from build123d import *

# Parameters (mm, degrees)
SKETCH2_W                    = 80
SKETCH2_H                    = 41
BOSS_EXTRUDE1_DEPTH          = 68
FILLET1_R                    = 3
SKETCH5_OUTSIDE_W            = 104.544
SKETCH5_OUTSIDE_H            = 65.544
CUT_EXTRUDE2_DEPTH           = 48
CUT_EXTRUDE3_DEPTH           = 82.672987579
FILLET2_R                    = 3
FILLET3_R                    = 3
M10_TAPPED_HOLE1_D           = 8.5
M10_TAPPED_HOLE1_DEPTH       = 16.946342369
M10_TAPPED_HOLE1_CSINK_D     = 10.05
M10_TAPPED_HOLE1_CSINK_ANGLE = 90
M10_TAPPED_HOLE1_TIP         = 2.553657631


with BuildPart() as part:
    # Sketch2 → Boss-Extrude1 (new body)
    with BuildSketch(Plane(origin=(0, 0, 0), x_dir=(1, 0, 0), z_dir=(0, 1, 0))):
        with Locations((0, -0.63)):
            Rectangle(SKETCH2_W, SKETCH2_H)
    extrude(amount=-BOSS_EXTRUDE1_DEPTH)

    # Fillet1
    fillet1_edges = [part.edges().sort_by_distance(p)[0] for p in [
        (40, -34, 21.13),
        (-40, -34, 21.13),
        (-40, -34, -19.87),
        (40, -34, -19.87),
    ]]
    fillet(fillet1_edges, radius=FILLET1_R)

    # Sketch5 outside → Cut-Extrude2 (cut)
    with BuildSketch(Plane.XZ.offset(68)):
        with Locations((0, 0.63)):
            Rectangle(SKETCH5_OUTSIDE_W, SKETCH5_OUTSIDE_H)
        with BuildLine():
            Line((19, -19.87), (24, -19.87))
            Line((24, -19.87), (24, 21.13))
            Line((24, 21.13), (-24, 21.13))
            Line((-24, 21.13), (-24, -19.87))
            Line((-24, -19.87), (-19, -19.87))
            Line((-19, -19.87), (-19, -14.37))
            ThreePointArc((-19, -14.37), (-17.242640687, -10.127359313), (-13, -8.37))
            Line((-13, -8.37), (-9, -8.37))
            ThreePointArc((-9, -8.37), (-6.878679656, -7.491320344), (-6, -5.37))
            Line((-6, -5.37), (-6, 10.13))
            ThreePointArc((-6, 10.13), (0, 16.13), (6, 10.13))
            Line((6, 10.13), (6, -5.37))
            ThreePointArc((6, -5.37), (6.878679656, -7.491320344), (9, -8.37))
            Line((9, -8.37), (13, -8.37))
            ThreePointArc((13, -8.37), (17.242640687, -10.127359313), (19, -14.37))
            Line((19, -14.37), (19, -19.87))
        make_face(mode=Mode.SUBTRACT)
    extrude(amount=-CUT_EXTRUDE2_DEPTH, mode=Mode.SUBTRACT)

    # Sketch6 → Cut-Extrude3 (cut, through all)
    with BuildSketch(Plane.XZ.offset(68)):
        with BuildLine():
            Line((-13, -8.37), (-9, -8.37))
            ThreePointArc((-9, -8.37), (-6.878679656, -7.491320344), (-6, -5.37))
            Line((-6, -5.37), (-6, 10.13))
            ThreePointArc((-6, 10.13), (0, 16.13), (6, 10.13))
            Line((6, 10.13), (6, -5.37))
            ThreePointArc((6, -5.37), (6.878679656, -7.491320344), (9, -8.37))
            Line((9, -8.37), (13, -8.37))
            ThreePointArc((13, -8.37), (17.242640687, -10.127359313), (19, -14.37))
            Line((19, -14.37), (19, -19.87))
            Line((19, -19.87), (-19, -19.87))
            Line((-19, -19.87), (-19, -14.37))
            ThreePointArc((-19, -14.37), (-17.242640687, -10.127359313), (-13, -8.37))
        make_face()
    extrude(amount=-CUT_EXTRUDE3_DEPTH, mode=Mode.SUBTRACT)

    # Fillet2
    fillet2_edges = [part.edges().sort_by_distance(p)[0] for p in [
        (24, -44, 21.13),
        (-24, -44, 21.13),
    ]]
    fillet(fillet2_edges, radius=FILLET2_R)

    # Fillet3
    # the kernel refuses this fillet: 3 mm, written as the material it adds along each edge
    with BuildSketch(Plane(origin=(24, -20, -19.87), x_dir=(0, -1, 0), z_dir=(0, 0, 1)), Plane(origin=(-24, -20, 18.13), x_dir=(0, -1, 0), z_dir=(0, 0, -1))) as fillet3_piece_1:
        with BuildLine():
            CenterArc((FILLET3_R, FILLET3_R), FILLET3_R, 180, 90)
            Line((0, FILLET3_R), (0, 0))
            Line((0, 0), (FILLET3_R, 0))
        make_face()
    extrude(amount=38)
    with BuildSketch(Plane(origin=(-21, -20, 18.13), x_dir=(0.5976672776328279, 0, -0.801744239297648), z_dir=(-0.801744239297648, 0, -0.5976672776328279))) as fillet3_piece_2_section:
        with BuildLine():
            CenterArc((3 + FILLET3_R, FILLET3_R), FILLET3_R, 180, 90)
            Line((3 + FILLET3_R, 0), (3, 0))
            Line((3, 0), (3, FILLET3_R))
        make_face()
    fillet3_piece_2 = revolve(axis=Axis((-21, -20, 18.13), (0, -1, 0)), revolution_arc=233.296989237, mode=Mode.PRIVATE)
    fillet3_piece_2 = split(fillet3_piece_2, bisect_by=Plane(origin=(-23.249816778, -20.934885373, 21.13), z_dir=(0, 0, -1)), keep=Keep.TOP, mode=Mode.PRIVATE)
    add(fillet3_piece_2)
    with BuildSketch(Plane(origin=(21, -20, 18.13), x_dir=(-0.5976672776328279, 0, -0.801744239297648), z_dir=(0.801744239297648, 0, -0.5976672776328279))) as fillet3_piece_3_section:
        with BuildLine():
            CenterArc((3 + FILLET3_R, -FILLET3_R), FILLET3_R, 90, 90)
            Line((3, -FILLET3_R), (3, 0))
            Line((3, 0), (3 + FILLET3_R, 0))
        make_face()
    fillet3_piece_3 = revolve(axis=Axis((21, -20, 18.13), (0, 1, 0)), revolution_arc=233.296989237, mode=Mode.PRIVATE)
    fillet3_piece_3 = split(fillet3_piece_3, bisect_by=Plane(origin=(23.249816872, -20.934884795, 21.13), z_dir=(0, 0, -1)), keep=Keep.TOP, mode=Mode.PRIVATE)
    add(fillet3_piece_3)

    # M10 Tapped Hole1
    with Locations(Plane(origin=(0, 0, 0), x_dir=(1, 0, 0), z_dir=(0, 1, 0))):
        with Locations((27.5, -0.63), (-27.5, -0.63)):
            CounterSinkHole(M10_TAPPED_HOLE1_D / 2, M10_TAPPED_HOLE1_CSINK_D / 2, depth=M10_TAPPED_HOLE1_DEPTH, counter_sink_angle=M10_TAPPED_HOLE1_CSINK_ANGLE)
            with Locations((0, 0, -(M10_TAPPED_HOLE1_DEPTH + M10_TAPPED_HOLE1_TIP / 2))):  # 118° drill point
                Cone(0, M10_TAPPED_HOLE1_D / 2, M10_TAPPED_HOLE1_TIP, mode=Mode.SUBTRACT)


solid = part.part
Check sheet for the modelled part. Datum: model origin and axes. Units: mm. A direction names the side the tool comes from. Round coordinates to 2 decimals unless told otherwise and drop trailing zeros. Write each loop counter-clockwise with the first axis right and the second up, starting at its lowest first coordinate (ties: lowest second). Pieces come first, ordered by that corner, then holes. Notation, with made-up numbers: (-39.75, 62) - (-4.75, 62) arc R13 cw to (-4.75, 73) - close; hole circle Ø10 at (13.5, -26.75). An arc over 180 degrees is marked (long way). Return JSON: item names as keys, results as strings.
Q1. Scan lines: L1, parallel to Z at x = 27.5, y = -6; L2, parallel to X at y = -39.5, z = 4; L3, parallel to X at y = -3.5, z = -15. Record each from-to range of solid material in increasing order. Write a range as from..to.
Returned:
{"L1": "z = -19.87..-3.62, 4.88..21.13", "L2": "x = -24..-6, 6..24", "L3": "x = -40..-19, 19..40"}
Q2. Depth check by flat-ended pin: P1, Ø2, axis at x = 10.5, y = -50.5, coming from the -Z side; P2, Ø19, axis at y = -54, z = 2.5, coming from the +X side; P3, Ø3, axis at y = -32, z = 5.5, coming from the -X side. Enter the tip coordinate at first touch or a pass-through.
Returned:
{"P1": "stops at z = -8.37", "P2": "stops at x = 24", "P3": "stops at x = -24"}
Q3. Cross-section at C-C (y = -43.5). Record the boundary of the cut face in (x, z).
Returned:
{"outline": "(-24, -19.87) - (-19, -19.87) - (-19, -14.37) arc R6 cw to (-13, -8.37) - (-9, -8.37) arc R3 ccw to (-6, -5.37) - (-6, 10.13) arc R6 cw to (6, 10.13) - (6, -5.37) arc R3 ccw to (9, -8.37) - (13, -8.37) arc R6 cw to (19, -14.37) - (19, -19.87) - (24, -19.87) - (24, 18.13) arc R3 ccw to (21, 21.13) - (-21, 21.13) arc R3 ccw to (-24, 18.13) - close"}
Q4. Draft check along X on faces 1 (the cylindrical face through (-24.9, -20.86, -0.6)), 2 (the cylindrical face through (23.1, -45.18, 20.27)), 3 (the cylindrical face through (-23.254, -8.974, 0.443)), 4 (the cylindrical face through (-0.13, -34.48, 16.13)). Enter one of: released by +X, released by -X, zero draft, split by the parting line, or undercut.
Returned:
{"face 1": "released by -X", "face 2": "released by +X", "face 3": "undercut", "face 4": "undercut"}
Q5. Cross-section at D-D (x = 11). Record the boundary of the cut face in (y, z).
Returned:
{"outline": "(-68, -8.37) - (0, -8.37) - (0, 21.13) - (-68, 21.13) - close"}
Q6. Cross-section at A-A (z = 7). Record the boundary of the cut face in (x, y).
Returned:
{"outline": "(-40, -20) - (-27, -20) arc R3 cw to (-24, -23) - (-24, -68) - (-6, -68) - (-6, 0) - (-40, 0) - close; (6, -68) - (24, -68) - (24, -23) arc R3 cw to (27, -20) - (40, -20) - (40, 0) - (6, 0) - close"}
Q7. Cross-section at B-B (y = -8). Record the boundary of the cut face in (x, z), then the cut area to 3 significant figures.
Returned:
{"outline": "(-40, -16.87) arc R3 ccw to (-37, -19.87) - (-19, -19.87) - (-19, -14.37) arc R6 cw to (-13, -8.37) - (-9, -8.37) arc R3 ccw to (-6, -5.37) - (-6, 10.13) arc R6 cw to (6, 10.13) - (6, -5.37) arc R3 ccw to (9, -8.37) - (13, -8.37) arc R6 cw to (19, -14.37) - (19, -19.87) - (37, -19.87) arc R3 ccw to (40, -16.87) - (40, 18.13) arc R3 ccw to (37, 21.13) - (-37, 21.13) arc R3 ccw to (-40, 18.13) - close; hole circle Ø8.5 at (-27.5, 0.63); hole circle Ø8.5 at (27.5, 0.63)", "area": "2,450 mm²"}
Q8. Access from +Z, -Z, +X, -X, +Y, -Y to the whole of each face (thin tool, end or side, straight path). Record for faces 5 (the cylindrical face through (6.86, -34.48, -7.47)), 6 (the flat face through (40, -10, 1)), 7 (the flat face through (-33, -20, 1)), 8 (the flat face through (24, -46, -1)).
Returned:
{"face 5": "-Z, +Y, -Y", "face 6": "+Z, -Z, +X, +Y, -Y", "face 7": "+Z, -Z, -X, -Y", "face 8": "+Z, -Z, +X, -Y"}
